Read the model definition and answer for the solid it produces. Units are mm, in the model's axes. Round coordinates to 2 decimals unless told otherwise and drop trailing zeros. Write each loop counter-clockwise with the first axis right and the second up, starting at its lowest first coordinate (ties: lowest second). Pieces come first, ordered by that corner, then holes. Notation, with made-up numbers: (-37.5, 26.5) - (-4.5, 26.5) arc R11 ccw to (-4.5, 35.5) - close; hole circle Ø1 at (-29, 85.5). An arc over 180 degrees is marked (long way). Answer as CSV lines item,"result". Start each with the question number.
1) Find section C-C on z = 5.5. Determine the outline of the cut face in (x, y).
2) Consider line 1 along X through (y, z) = (-4, 3.75); line 2 along X through (y, z) = (44.5, 5.5); line 3 along Y through (x, z) = (13.5, 1.5). Determine where each line is inside the solid, lowest interval first.
3) Each of these flat-tipped pins is pushed along its axis until it touches: pin 1 (5 mm diameter, centred on y = 27, z = 8, fed in from -X); pin 2 (1.5 mm diameter, centred on y = -11.5, z = 2, fed in from +X); pin 3 (4 mm diameter, centred on x = 31.5, z = 4, fed in from -Y). Where does it stop, or does it pass through?
from build123d import *

# Parameters (mm, degrees)
F0_W     = 103.053610972
F0_H     = 103.053610972
F1_DEPTH = 10
F2_SIZE2 = 3.42161
F2_SIZE  = 9.99999
F3_SIZE2 = 3.42161
F3_SIZE  = 9.99999
F4_SIZE2 = 3.42161
F4_SIZE  = 9.99999
F5_SIZE2 = 3.42161
F5_SIZE  = 9.99999


# Not quite as in the source:
# - a fillet or chamfer is up to 0.001 mm smaller than in the source, because OpenCascade refuses the exact size


with BuildPart() as f1:
    # F0 (on Top) → F1 (new body)
    with BuildSketch(Plane.XY):
        with Locations((-4.9147187663, 3.5890949971)):
            Rectangle(F0_W, F0_H)
    extrude(amount=F1_DEPTH)

    # F2 (size 10 and 3.421620486 in the source; OpenCascade refuses exactly that, so slightly less here)
    f2_edges = [f1.edges().sort_by_distance(p)[0] for p in [
        (46.612087, 3.589095, 10),
    ]]
    f2_side = f1.faces().sort_by_distance((46.612087, 3.589095, 5))[0]
    chamfer(f2_edges, length=F2_SIZE, length2=F2_SIZE2, reference=f2_side)

    # F3 (size 10 and 3.421620486 in the source; OpenCascade refuses exactly that, so slightly less here)
    f3_edges = [f1.edges().sort_by_distance(p)[0] for p in [
        (-6.625524, 55.1159, 10),
    ]]
    f3_side = f1.faces().sort_by_distance((-5.765307, 55.1159, 4.971864))[0]
    chamfer(f3_edges, length=F3_SIZE, length2=F3_SIZE2, reference=f3_side)

    # F4 (size 10 and 3.421620486 in the source; OpenCascade refuses exactly that, so slightly less here)
    f4_edges = [f1.edges().sort_by_distance(p)[0] for p in [
        (-6.625524, -47.93771, 10),
    ]]
    f4_side = f1.faces().sort_by_distance((-5.765307, -47.93771, 4.971864))[0]
    chamfer(f4_edges, length=F4_SIZE, length2=F4_SIZE2, reference=f4_side)

    # F5 (size 10 and 3.421620486 in the source; OpenCascade refuses exactly that, so slightly less here)
    f5_edges = [f1.edges().sort_by_distance(p)[0] for p in [
        (-56.441524, 3.589095, 10),
    ]]
    f5_side = f1.faces().sort_by_distance((-56.441524, 3.589095, 4.942762))[0]
    chamfer(f5_edges, length=F5_SIZE, length2=F5_SIZE2, reference=f5_side)


solid = f1.part
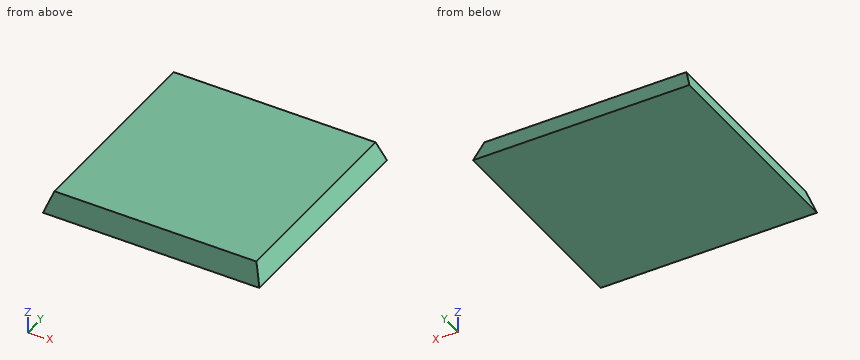
Check values:
1,outline,"(-54.56, -46.06) - (44.73, -46.06) - (44.73, 53.23) - (-54.56, 53.23) - close"
2,line 1,"x = -55.16 to 45.33"
2,line 2,"x = -54.56 to 44.73"
2,line 3,"y = -47.42 to 54.6"
3,pin 1,"stops at x = -54.56"
3,pin 2,"stops at x = 46.18"
3,pin 3,"stops at y = -47.25"
